Design review of the part built by this model. Coordinates are the model's own, in mm. Coordinates: 2 decimals unless noted, no trailing zeros. Loops run counter-clockwise (first coordinate to the right, second up) from the corner with the lowest first, then second, coordinate; pieces in that order, holes last.
Q1. For P1, Ø4, axis at x = 23, y = 16, coming from the +Z side; P2, Ø12, axis at x = -6, z = -13.5, coming from the +Y side; P3, Ø10, axis at x = -16, z = -1.5, coming from the +Y side, all flat-tipped, find the tip position at first contact; note any pin that passes through.
Q2. Draft analysis for pull direction Z (two halves, no side actions). For faces 1 (the face through (0.6, 29.449, -18.775)), 2 (the face through (-42.862, -31, -17)), 3 (the face through (0.6, 37.776, 4.96)), state which applies: released by +Z, released by -Z, zero draft, split by the parting line, or undercut.
Q3. Add section C-C on x = 4. Give the boundary of the cut face in (y, z) (3 decimals), and give its area (3 significant figures).
Q4. Add section D-D on x = -32. Give the boundary of the cut face in (y, z) (3 decimals), and give its area (3 significant figures).
Q5. Add section A-A on y = 0. Give the boundary of the cut face in (x, z) (1 decimal), and give its area (3 significant figures).
Q6. Wall thickness on probe 1 along Y at (x, z) = (-22, -9); probe 2 along Y at (x, z) = (-2, 0) (3 decimals); probe 3 along Z at (x, y) = (-36, -5.5): over which ranges is each line inside the solid? List them lowest first.
Q7. Add section B-B on z = -7. Give the boundary of the cut face in (x, y).
```python
from build123d import *

# Parameters (mm, degrees)
SKETCH1_R               = 38.1
BOSS_EXTRUDE1_DEPTH     = 42.8625
SHELL1_T                = -3.175
CUT_EXTRUDE1_DEPTH      = 69.850663804
CUT_EXTRUDE1_DEPTH_BACK = 69.850663804
SKETCH2_R               = 25.4


with BuildPart() as part:
    # Sketch1 → Boss-Extrude1 (new, symmetric)
    with BuildSketch(Plane(origin=(0, 0, 0), x_dir=(0, 0, -1), z_dir=(1, 0, 0))):
        Circle(SKETCH1_R)
    extrude(amount=BOSS_EXTRUDE1_DEPTH, both=True)

    # Shell1
    shell1_openings = [part.faces().sort_by_distance(p)[0] for p in [
        (42.8625, 0, 0),
        (-42.8625, 0, 0),
    ]]
    offset(amount=SHELL1_T, openings=shell1_openings, kind=Kind.INTERSECTION)

    # Sketch2 → Cut-Extrude1 (cut, two sides: drawn at the far end of the back side and taken through both)
    with BuildSketch(Plane.XY.offset(-CUT_EXTRUDE1_DEPTH_BACK)):
        with Locations(Location((-3.96875, 0, 0), (0, 0, 180))):
            Circle(SKETCH2_R)
    extrude(amount=CUT_EXTRUDE1_DEPTH + CUT_EXTRUDE1_DEPTH_BACK, mode=Mode.SUBTRACT)


solid = part.part
```
Entries:
1. P1: stops at z = 35.43
1. P2: stops at y = 37.35
1. P3: stops at y = 38.1
2. face 1: undercut
2. face 2: zero draft
2. face 3: split by the parting line
3. outline: (-24.118, -29.495) - (-24.118, -25.261) arc R34.925 cw to (-24.118, 25.261) - (-24.118, 29.495) arc R38.1 ccw to start; (24.118, -29.495) arc R38.1 ccw to (24.118, 29.495) - (24.118, 25.261) arc R34.925 cw to (24.118, -25.261) - close
3. area: 394 mm2
4. outline: circle Ø76.2 at (0, 0); hole circle Ø69.85 at (0, 0)
4. area: 728 mm2
5. outline: (-42.9, -38.1) - (-29.4, -38.1) - (-29.4, -34.9) - (-42.9, -34.9) - close; (-42.9, 34.9) - (-29.4, 34.9) - (-29.4, 38.1) - (-42.9, 38.1) - close; (21.4, -38.1) - (42.9, -38.1) - (42.9, -34.9) - (21.4, -34.9) - close; (21.4, 34.9) - (42.9, 34.9) - (42.9, 38.1) - (21.4, 38.1) - close
5. area: 222 mm2
6. probe 1: y = -37.02 to -33.75, 33.75 to 37.02
6. probe 2: y = -38.1 to -34.925, 34.925 to 38.1
6. probe 3: z = -37.7 to -34.49, 34.49 to 37.7
7. outline: (-42.86, -37.45) - (42.86, -37.45) - (42.86, -34.22) - (-42.86, -34.22) - close; (-42.86, 34.22) - (42.86, 34.22) - (42.86, 37.45) - (-42.86, 37.45) - close
